from build123d import *


with BuildPart() as f2:
    # F2: sweep along a path in F0
    with BuildLine(Plane.XY) as f2_path:
        CenterArc((0, 0), 30.1625, 0, 360)
    # F1 (on Front) → F2 (sweep)
    with BuildSketch(Plane.XZ):
        Polygon((26.87468, -7.9375), (33.45032, -7.9375), (38.1, -3.28782), (38.1, 3.28782), (33.45032, 7.9375), (26.87468, 7.9375), (22.225, 3.28782), (22.225, -3.28782), align=None)
    sweep(path=f2_path.line)


solid = f2.part
Design review of the part built by this model. Coordinates are the model's own, in mm. Coordinates: 2 decimals unless noted, no trailing zeros. Use one line per item in the form item = value.
(1) Draft analysis for pull direction X (two halves, no side actions). For faces 1 (the face through (-4.867, -21.917, 3.514)), 2 (the face through (-30.235, -23.183, 0.046)), 3 (the face through (21.199, 6.676, -0.046)), state which applies: pulls with the +X half, pulls with the -X half, needs draft (parallel to the pull), parting line crosses it, or undercut.
Return value:
face_1 = undercut
face_2 = parting line crosses it
face_3 = undercut
(2) For line 1 along Y through (x, z) = (0, -1.5) (3 decimals); line 2 along Y through (x, z) = (-27, -2.5); line 3 along X through (y, z) = (1, -2), list the stretches that pass through material, from the lowest coordinate up. Write a range as from..to.
Return value:
line_1 = -38.1..-22.225, 22.225..38.1
line_2 = -26.88..26.88
line_3 = -38.09..-22.2, 22.2..38.09
(3) Clearance check with flat-ended pins moving along their axes: P1, Ø2, axis at x = -10.5, y = 19.5, coming from the +Z side; P2, Ø6, axis at y = 17, z = 4.5, coming from the -X side; P3, Ø3, axis at x = -18.5, z = 6.5, coming from the +Y side. State where each tip first meets the part, or that it passes through.
Return value:
P1 = 4.21
P2 = -35.33
P3 = 31.54
